from build123d import *

# Parameters (mm, degrees)
F0_W     = 30
F0_H     = 30
F1_DEPTH = 30
F2_R     = 5
F3_DEPTH = 30
F4_R     = 5.7203
F5_DEPTH = 30


with BuildPart() as f1:
    # F0 (on Front) → F1 (new body)
    with BuildSketch(Plane.XZ):
        Rectangle(F0_W, F0_H)
    extrude(amount=-F1_DEPTH)

    # F2 (on face) → F3 (cut)
    with BuildSketch(Plane.XZ):
        Circle(F2_R)
    extrude(amount=-F3_DEPTH, mode=Mode.SUBTRACT)

    # F4 (on face) → F5 (join)
    with BuildSketch(Plane.XY.offset(15)):
        with Locations((0, 15.874371)):
            Circle(F4_R)
    extrude(amount=F5_DEPTH)


solid = f1.part
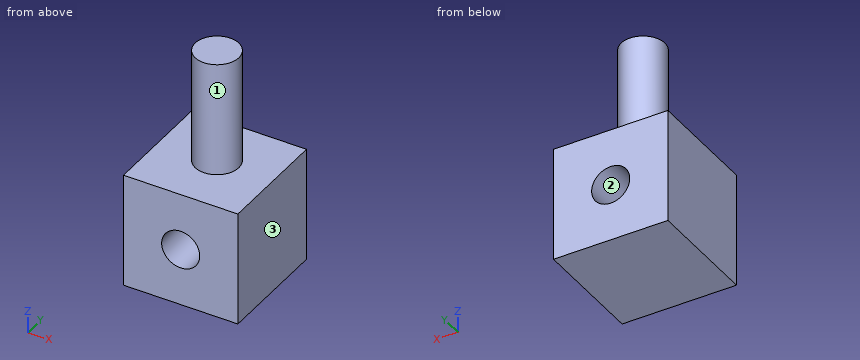
Input: part model. Units: mm. Frame: model coordinates. Face numbers are marked on the shaded views. Give positions to 0.01 mm unless a question says otherwise; leave off trailing zeros. Loops run counter-clockwise (first coordinate to the right, second up) from the corner with the lowest first, then second, coordinate; pieces in that order, holes last. Notation, with made-up numbers: (34.5, 56.25) - (54.5, 56.25) arc R11 ccw to (54.5, 63.25) - close; hole circle Ø7 at (-38.75, 70.5). An arc over 180 degrees is marked (long way). Use CSV: the item, a comma, the result in double quotes. Start each with the question number.
Item 1: Section D-D on x = 3.5. Return loops of the section in (y, z), then the cut area to 3 significant figures.
Item 2: Contact query for flat-ended pins moving along their axis: P1, Ø5, axis at y = 11.5, z = 31.5, coming from the +X side; P2, Ø5, axis at x = -6.5, y = 27, coming from the +Z side. Output: stop coordinate, or through.
Item 3: Mould query, pull axis X, two halves, no side actions, for the marked faces 1, 2 and 3. Classes: pulls with the +X half, pulls with the -X half, needs draft (parallel to the pull), parting line crosses it, or undercut.
Item 4: Section C-C on y = 2. Return loops of the section in (x, z).
Item 5: Section B-B on z = 0. Return loops of the section in (x, y).
Item 6: Line query: line 1 (Z direction, x = 0, y = 9.75); line 2 (Z direction, x = 0, y = 14.25); line 3 (Z direction, x = 7.75, y = 19). Output: solid intervals per line, ascending.
Item 7: Section A-A on x = 0. Return loops of the section in (y, z), then the cut area to 3 significant figures.
Ans:
1,outline,"(0, -15) - (30, -15) - (30, -3.57) - (0, -3.57) - close; (0, 3.57) - (30, 3.57) - (30, 15) - (20.4, 15) - (20.4, 45) - (11.35, 45) - (11.35, 15) - (0, 15) - close"
1,area,"957 mm2"
2,P1,"stops at x = 5.4"
2,P2,"stops at z = 15"
3,face 1,"parting line crosses it"
3,face 2,"undercut"
3,face 3,"pulls with the +X half"
4,outline,"(-15, -15) - (15, -15) - (15, 15) - (-15, 15) - close; hole circle Ø10 at (0, 0)"
5,outline,"(-15, 0) - (-5, 0) - (-5, 30) - (-15, 30) - close; (5, 0) - (15, 0) - (15, 30) - (5, 30) - close"
6,line 1,"z = -15 to -5, 5 to 15"
6,line 2,"z = -15 to -5, 5 to 45"
6,line 3,"z = -15 to 15"
7,outline,"(0, -15) - (30, -15) - (30, -5) - (0, -5) - close; (0, 5) - (30, 5) - (30, 15) - (21.59, 15) - (21.59, 45) - (10.15, 45) - (10.15, 15) - (0, 15) - close"
7,area,"943 mm2"
